Autodesk Inventor part; units mm, degrees
ref_plane "YZ Plane" through (0, 0, 0) normal (1, 0, 0) x (0, 1, 0)
ref_plane "XZ Plane" through (0, 0, 0) normal (0, 1, 0) x (-1, 0, 0)
ref_plane "XY Plane" through (0, 0, 0) normal (0, 0, 1) x (1, 0, 0)
sketch "Sketch1" plane through (0, 0, 0) normal (1, 0, 0) x (0, 1, 0)
  circle A0 centre (0, -124) radius 1.95
  circle A1 centre (0, 124) radius 1.95
  circle A2 centre (-19, -65) radius 1.5
  circle A3 centre (-19, 65) radius 1.5
  line L0 (0, 124) -> (-19, 65) construction
  line L1 (4.7593, 122.4673) -> (-14.2407, 63.4673)
  line L2 (-23.7593, 66.5327) -> (-4.7593, 125.5327)
  arc A4 (4.7593, 122.4673) -> (-4.7593, 125.5327) centre (0, 124) ccw
  arc A5 (-23.7593, 66.5327) -> (-14.2407, 63.4673) centre (-19, 65) ccw
  line L3 (-19, 65) -> (-19, -65) construction
  line L4 (-24, 65) -> (-24, -65)
  line L5 (-14, -65) -> (-14, 65)
  arc A6 (-14, 65) -> (-24, 65) centre (-19, 65) ccw
  arc A7 (-24, -65) -> (-14, -65) centre (-19, -65) ccw
  line L6 (-19, -65) -> (0, -124) construction
  line L7 (-23.7593, -66.5327) -> (-4.7593, -125.5327)
  line L8 (4.7593, -122.4673) -> (-14.2407, -63.4673)
  arc A8 (-14.2407, -63.4673) -> (-23.7593, -66.5327) centre (-19, -65) ccw
  arc A9 (-4.7593, -125.5327) -> (4.7593, -122.4673) centre (0, -124) ccw
  circle A10 centre (-44, 65) radius 1.5
  circle A11 centre (-44, -65) radius 1.5
  line L9 (-19, 65) -> (-44, 65) construction
  line L10 (-19, 67) -> (-44, 67)
  line L11 (-44, 63) -> (-19, 63)
  arc A12 (-19, 63) -> (-19, 67) centre (-19, 65) ccw
  arc A13 (-44, 67) -> (-44, 63) centre (-44, 65) ccw
  line L12 (-19, -65) -> (-44, -65) construction
  line L13 (-19, -63) -> (-44, -63)
  line L14 (-44, -67) -> (-19, -67)
  arc A14 (-19, -67) -> (-19, -63) centre (-19, -65) ccw
  arc A15 (-44, -63) -> (-44, -67) centre (-44, -65) ccw
  line L15 (0, 124) -> (-44, 65) construction
  line L16 (-4.0081, 126.9891) -> (-48.0081, 67.9891)
  line L17 (-39.9919, 62.0109) -> (4.0081, 121.0109)
  arc A16 (4.0081, 121.0109) -> (-4.0081, 126.9891) centre (0, 124) ccw
  arc A17 (-48.0081, 67.9891) -> (-39.9919, 62.0109) centre (-44, 65) ccw
  line L18 (-44, -65) -> (0, -124) construction
  line L19 (-48.0081, -67.9891) -> (-4.0081, -126.9891)
  line L20 (4.0081, -121.0109) -> (-39.9919, -62.0109)
  arc A18 (-39.9919, -62.0109) -> (-48.0081, -67.9891) centre (-44, -65) ccw
  arc A19 (-4.0081, -126.9891) -> (4.0081, -121.0109) centre (0, -124) ccw
  line L21 (-44, 65) -> (-44, -65) construction
  line L22 (-49, 65) -> (-49, -65)
  line L23 (-39, -65) -> (-39, 65)
  arc A20 (-39, 65) -> (-49, 65) centre (-44, 65) ccw
  arc A21 (-49, -65) -> (-39, -65) centre (-44, -65) ccw
  line L24 (-44, 65) -> (-19, 0) construction
  line L25 (-45.4, 64.4615) -> (-20.4, -0.5385)
  line L26 (-17.6, 0.5385) -> (-42.6, 65.5385)
  arc A22 (-42.6, 65.5385) -> (-45.4, 64.4615) centre (-44, 65) ccw
  arc A23 (-20.4, -0.5385) -> (-17.6, 0.5385) centre (-19, 0) ccw
  line L27 (-44, -65) -> (-19, 0) construction
  line L28 (-42.6, -65.5385) -> (-17.6, -0.5385)
  line L29 (-20.4, 0.5385) -> (-45.4, -64.4615)
  arc A24 (-45.4, -64.4615) -> (-42.6, -65.5385) centre (-44, -65) ccw
  arc A25 (-17.6, -0.5385) -> (-20.4, 0.5385) centre (-19, 0) ccw
  line L30 (-19, 0) -> (-44, 0) construction
  line L31 (-19, 1.5) -> (-44, 1.5)
  line L32 (-44, -1.5) -> (-19, -1.5)
  arc A26 (-19, -1.5) -> (-19, 1.5) centre (-19, 0) ccw
  arc A27 (-44, 1.5) -> (-44, -1.5) centre (-44, 0) ccw
  circle A28 centre (-19, -10) radius 1.5
  circle A29 centre (-19, -35) radius 1.5
  circle A30 centre (-19, 10) radius 1.5
  circle A31 centre (-19, 35) radius 1.5
  circle A32 centre (0, -124) radius 12.5
  circle A33 centre (0, 124) radius 12.5
  circle A34 centre (-22, 94.5) radius 1.5
  circle A35 centre (-22, -94.5) radius 1.5
  circle A36 centre (-11.3392, 88.7888) radius 1.5
  circle A37 centre (-11.3392, -88.7888) radius 1.5
  circle A38 centre (-11.3392, 88.7888) radius 5
  circle A39 centre (-22, 94.5) radius 5
  circle A40 centre (-11.3392, -88.7888) radius 5
  circle A41 centre (-22, -94.5) radius 5
  circle A42 centre (-19, 65) radius 4
  circle A43 centre (-44, 65) radius 4
  circle A44 centre (-19, -65) radius 4
  circle A45 centre (-44, -65) radius 4
  circle A46 centre (-19, 0) radius 1
  line L33 (-22, 94.5) -> (-11.3392, 88.7888) construction
  line L34 (-24.3611, 90.0926) -> (-13.7003, 84.3814)
  line L35 (-8.9781, 93.1962) -> (-19.6389, 98.9074)
  arc A47 (-19.6389, 98.9074) -> (-24.3611, 90.0926) centre (-22, 94.5) ccw
  arc A48 (-13.7003, 84.3814) -> (-8.9781, 93.1962) centre (-11.3392, 88.7888) ccw
  line L36 (-11.3392, -88.7888) -> (-22, -94.5) construction
  line L37 (-13.7003, -84.3814) -> (-24.3611, -90.0926)
  line L38 (-19.6389, -98.9074) -> (-8.9781, -93.1962)
  arc A49 (-8.9781, -93.1962) -> (-13.7003, -84.3814) centre (-11.3392, -88.7888) ccw
  arc A50 (-24.3611, -90.0926) -> (-19.6389, -98.9074) centre (-22, -94.5) ccw
  circle A51 centre (0, -124) radius 15
  circle A52 centre (0, 124) radius 15
  point P0 (0, 0)
  point P1 (-9.5, 94.5)
  point P2 (-9.5, -94.5)
  point P3 (-14, -64.2148)
  point P4 (-14, 64.2148)
  point P5 (-24, 65)
  point P6 (-23.7593, -66.5327)
  point P7 (-31.5, 65)
  point P8 (-31.5, -65)
  point P9 (-44, 0)
  point P10 (-31.5, 32.5)
  point P11 (-31.5, -32.5)
  point P12 (-39, 47.8215)
  point P13 (-24, 8.8215)
  point P14 (-24, 17.1785)
  point P15 (-41.6236, 63)
  point P16 (-24, 63)
  point P17 (-23.6088, 67)
  point P18 (-36.2712, 67)
  point P19 (-13.9854, 96.8832)
  point P20 (-6.8749, 118.9633)
  point P21 (-43.3898, 70)
  point P22 (-46.5, 65)
  point P23 (-46.5, -65)
  point P24 (-43.3898, -70)
  point P25 (-6.8749, -118.9633)
  point P26 (-13.9854, -96.8832)
  point P27 (-36.2712, -67)
  point P28 (-23.6088, -67)
  point P29 (-24, -63)
  point P30 (-41.6236, -63)
  point P31 (-24, -17.1785)
  point P32 (-24, -8.8215)
  point P33 (-39, -47.8215)
  point P34 (-31.5, 0)
  point P35 (-39, -1.5)
  point P36 (-24, -1.5)
  point P37 (-24, 1.5)
  point P38 (-39, 1.5)
  point P39 (-49, -65)
  point P40 (-24, -65)
  point P41 (-4.0081, -126.9891)
  point P42 (-4.0081, 126.9891)
  point P43 (-14.2407, -63.4673)
  point P44 (-4.0081, 126.9891)
  point P45 (-14.2407, 63.4673)
  point P46 (4.7593, 122.4673)
  point P47 (-14.2407, -63.4673)
  point P48 (-39, 63)
  point P49 (-23.5826, 67)
  point P50 (-14, 65)
  point P51 (-39, -63)
  point P52 (-39, -56.1785)
  point P53 (-39, 56.1785)
  point P54 (-10.8571, -117.8053)
  point P55 (1.2475, -111.5624)
  point P56 (-10.8571, 117.8053)
  point P57 (1.2475, 111.5624)
  point P58 (-40.8878, -61.0867)
  point P59 (-41.5, 60.6699)
  point P60 (-23.7593, 66.5327)
  point P61 (-16.0985, -90.3215)
  point P62 (-6.5799, -87.2562)
  point P63 (-6.5799, 87.2562)
  point P64 (-16.0985, 90.3215)
  point P65 (-17.9919, 91.5109)
  point P66 (-26.0081, 97.4891)
  point P67 (-26.0081, -97.4891)
  point P68 (-17.9919, -91.5109)
  point P69 (-16.5, -61.8775)
  point P70 (-15.6632, -67.2059)
  point P71 (-22.4641, -67)
  point P72 (-20.4225, -68.7385)
  point P73 (-21.5, -61.8775)
  point P74 (-22.4641, -63)
  point P75 (-40.5359, -63)
  point P76 (-41.2689, -62.0775)
  point P77 (-46.5, -61.8775)
  point P78 (-44.1374, -68.9976)
  point P79 (-41.2689, 62.0775)
  point P80 (-40.5359, 63)
  point P81 (-44.1374, 68.9976)
  point P82 (-46.5, 61.8775)
  point P83 (-22.4641, 63)
  point P84 (-21.5, 61.8775)
  point P85 (-20.4225, 68.7385)
  point P86 (-22.4641, 67)
  point P87 (-16.5, 61.8775)
  point P88 (-15.6632, 67.2059)
  point P89 (-16.6696, 91.6444)
  point P90 (-16.6696, -91.6444)
  point P91 (-19.6389, 98.9074)
  point P92 (-20.5658, 88.0594)
  point P93 (-17.3771, 86.3511)
  point P94 (-8.9781, 93.1962)
  point P95 (-8.9781, -93.1962)
  point P96 (-17.3771, -86.3511)
  point P97 (-20.5658, -88.0594)
  point P98 (-19.6389, -98.9074)
  point P99 (-24, -65)
  point P100 (-23.5826, -63)
  point P101 (-23.5826, -67)
  point P102 (-39, -63.3409)
  point P103 (-44.9251, 63.2268)
  point P104 (-39, 63.3409)
  point P105 (-23.5826, 63)
  point P106 (-24, 65)
  point P107 (-14.2613, -96.0265)
  point P108 (-14.2613, 96.0265)
  point P109 (-40.5359, 67)
  point P110 (-40.5359, -67)
  point P111 (0.4243, 109.006)
  point P112 (-12.4626, 115.6524)
  point P113 (-14.5206, 96.1655)
  point P114 (-12.4626, -115.6524)
  point P115 (0.4243, -109.006)
  point P116 (-14.5206, -96.1655)
  dimension "d2" = 3.9
  dimension "d4" = 3.9
  dimension "d25" = 3
  dimension "d28" = 3
  dimension "d43" = 59
  dimension "d44" = 65
  dimension "d45" = 65
  dimension "d47" = 59
  dimension "d48" = 10
  dimension "d49" = 10
  dimension "d50" = 10
  dimension "d53" = 3
  dimension "d54" = 3
  dimension "d55" = 4
  dimension "d56" = 4
  dimension "d57" = 25
  dimension "d58" = 25
  dimension "d59" = 10
  dimension "d60" = 10
  dimension "d61" = 10
  dimension "d62" = 3
  dimension "d63" = 3
  dimension "d64" = 3
  dimension "d65" = 3
  dimension "d66" = 3
  dimension "d67" = 10
  dimension "d68" = 25
  dimension "d69" = 3
  dimension "d70" = 3
  dimension "d71" = 10
  dimension "d72" = 25
  dimension "d73" = 25
  dimension "d74" = 25
  dimension "d76" = 3
  dimension "d78" = 3
  dimension "d79" = 3
  dimension "d80" = 3
  dimension "d81" = 6
  dimension "d82" = 6
  dimension "d83" = 19
  dimension "d84" = 8
  dimension "d85" = 8
  dimension "d86" = 8
  dimension "d87" = 8
  dimension "d88" = 2
  dimension "d89" = 10
  dimension "d90" = 10
  dimension "d91" = 30
  dimension "d92" = 30
extrude "Extrusion1" add sketch "Sketch1" along normal blind 5 contours L1 L5 A6 L10 L2 L34 A38 | A38 | L5 L8 A8 L13 L4 L28 A23 L26 L11 A5 L1 | L1 A5 L11 A42 L10 A6 L5 | L34 L2 A38 | A39 L34 L17 L10 A20 L16 | A39 | L8 A40 L37 L7 L14 A7 L5 | L5 A7 L14 A44 L13 A8 L8 | L2 L34 L17 L35 | L2 L35 A38 | L2 L10 L17 L34 | L17 A39 L35 | A20 L10 A43 L25 A17 | A39 L17 L34 | L11 L4 A5 | A5 A6 L10 A42 L11 | A40 | A6 L2 L10 | L2 A5 L4 L11 L23 L17 L10 | A17 L25 L23 L31 A27 L32 L29 A18 L22 | A20 L23 L17 L11 A43 L10 | L10 L17 L23 A20 | L4 L26 L23 L11 | A42 L10 A12 L11 | L11 A12 L10 A42 | L14 L7 A7 | A7 A8 L13 A44 L14 | A40 L7 L37 | A8 L4 L13 | L25 A43 L26 A17 | A17 L26 L23 L25 | A18 L29 A45 L14 A21 | A43 L11 L26 A10 L25 A13 L10 | L10 A13 L25 A43 | L26 A25 L31 L25 L4 | L4 L25 L23 L26 | L23 L26 A17 L17 L11 | L11 L17 L23 | L7 L14 L20 L23 L13 L4 A7 | L7 L37 L20 L14 | A44 L13 A14 L14 | L14 A14 L13 A44 | L38 L7 A40 | L7 L38 L20 L37 | L13 L23 L28 L4 | L26 A43 L11 L17 A17 | L25 A13 L11 L26 A43 | L25 L4 L31 L23 | A21 L14 L20 L37 A41 L19 | L29 L23 L28 A18 | A18 L28 A45 L29 | L25 L31 L4 | A23 L25 L29 A25 | L14 A21 L23 L20 | L20 A41 L37 | L28 L23 L29 L4 | L4 L29 L32 A23 L28 | L23 L20 L13 | L13 L20 A18 L28 L23 | L26 L11 A43 | L25 A10 L26 L11 A13 | L31 L4 L32 L23 | L23 L32 A27 L31 | A41 | L14 A45 L13 L20 L23 A21 | A18 L20 L13 A45 L28 | L23 L32 L4 L29 | A45 L28 L13 A15 L29 | L29 A15 L14 A45 | L31 L25 L29 L32 L4 | L31 A25 L29 L25 | L38 A41 L20 | L4 L32 L29 | L14 A15 L29 A11 L28 L13 A45 | A45 L13 L28 | A15 L13 L28 A11 L29 | L25 A23 L32 L29 | A46
sketch "Sketch8" plane through (5, 0, 0) normal (1, 0, 0) x (0, 0, -1)
  circle A0 centre (-94.5, -22) radius 1.5
  circle A1 centre (94.5, -22) radius 1.5
  line L0 (97.4891, -26.0081) -> (67.9891, -48.0081)
  line L1 (-67.9891, -48.0081) -> (-97.4891, -26.0081)
  arc A2 (65, -49) -> (67.9891, -48.0081) centre (65, -44) ccw
  line L2 (65, -49) -> (-65, -49)
  arc A3 (-67.9891, -48.0081) -> (-65, -49) centre (-65, -44) ccw
  line L3 (-87.2562, -6.5799) -> (-64.2148, -14)
  line L4 (-64.2148, -14) -> (64.2148, -14)
  line L5 (64.2148, -14) -> (87.2562, -6.5799)
  circle A4 centre (65, -44) radius 1.5
  circle A5 centre (-65, -19) radius 1.5
  circle A6 centre (65, -19) radius 1.5
  circle A7 centre (88.7888, -11.3392) radius 1.5
  circle A8 centre (-88.7888, -11.3392) radius 1.5
  circle A9 centre (-65, -44) radius 1.5
  arc A10 (-87.2562, -6.5799) -> (-93.1962, -8.9781) centre (-88.7888, -11.3392) ccw
  arc A11 (93.1962, -8.9781) -> (87.2562, -6.5799) centre (88.7888, -11.3392) ccw
  line L6 (93.1962, -8.9781) -> (98.9074, -19.6389)
  arc A12 (97.4891, -26.0081) -> (98.9074, -19.6389) centre (94.5, -22) ccw
  arc A13 (-98.9074, -19.6389) -> (-97.4891, -26.0081) centre (-94.5, -22) ccw
  line L7 (-98.9074, -19.6389) -> (-93.1962, -8.9781)
  circle A14 centre (10, -19) radius 1.5
  circle A15 centre (35, -19) radius 1.5
  circle A16 centre (-10, -19) radius 1.5
  circle A17 centre (-35, -19) radius 1.5
  point P0 (0, 0)
properties part number "Horizontal_bar_support_V2"
Design review of the part built by this model. Coordinates are the model's own, in mm. A direction names the side the tool comes from. Give positions to 0.01 mm unless a question says otherwise; leave off trailing zeros. Loops run counter-clockwise (first coordinate to the right, second up) from the corner with the lowest first, then second, coordinate; pieces in that order, holes last. Notation, with made-up numbers: (23, -0.75) - (57, -0.75) arc R15 cw to (57, 28.25) - close; hole circle Ø7 at (59, 80.25). An arc over 180 degrees is marked (long way). Use CSV: the item, a comma, the result in double quotes. Start each with the question number.
1. Add section A-A (x = 3.15). Count the separate pieces of the cut face and the enclosed holes in it, plus the area to 3 significant figures.
2. Wall thickness on L1, parallel to Z at x = 1.65, y = -44; L2, parallel to Y at x = 2.65, z = -0.5; L3, parallel to Y at x = 1.1, z = -64.5: over which ranges is each line inside the solid? List them lowest first.
3. Machinability: for faces 1 (the flat face through (2, -14, -1)), 2 (the cylindrical face through (2.5, -23, -99.4)), which of the approach directions +Z, -Z, +X, -X, +Y, -Y give a long, thin tool a straight path to every point of the face, cutting with its end or side? Answer none if there is none.
4. Add section C-C (y = -35). State the section outline as (x, z) points, plus the area to 3 significant figures.
5. Draft analysis for pull direction Z (two halves, no side actions). For faces 3 (the flat face through (2.465, -10.238, 75.897)), 4 (the flat face through (2.5, -14.4, -96.1)), 5 (the flat face through (5, -28, 1)), 6 (the flat face through (2.465, -10.238, -75.897)), state which applies: released by +Z, released by -Z, zero draft, split by the parting line, or undercut.
6. Insertion check: P1, Ø2.5, axis at y = -19, z = 35, coming from the -X side (3 decimals); P2, Ø1.5, axis at x = 3, y = -11, coming from the -Z side; P3, Ø3, axis at x = 2, y = -31.5, coming from the -Z side; P4, Ø2, axis at x = 2, y = -13.5, coming from the -Z side. Each pin has a flat end and moves straight along its axis. Give the tip position at first contact, or say it passes through.
7. Add section B-B (z = 15). State the section outline as (x, y) points, plus the area to 3 significant figures.
Results found:
1,separate pieces,"1"
1,enclosed holes,"12"
1,area,"6,320 mm²"
2,L1,"z = -73.36 to -66.5, -63.5 to 63.5, 66.5 to 73.36"
2,L2,"y = -49 to -14"
2,L3,"y = -49 to -45.41, -42.59 to -20.41, -17.59 to -13.91"
3,face 1,"+X, -X, +Y"
3,face 2,"-Z, +X, -X"
4,outline,"(0, -85.43) - (5, -85.43) - (5, 85.43) - (0, 85.43) - close"
4,area,"854 mm²"
5,face 3,"undercut"
5,face 4,"released by -Z"
5,face 5,"zero draft"
5,face 6,"undercut"
6,P1,"passes through"
6,P2,"stops at z = -94.68"
6,P3,"stops at z = -92.14"
6,P4,"stops at z = -96.15"
7,outline,"(0, -49) - (5, -49) - (5, -14) - (0, -14) - close"
7,area,"175 mm²"
